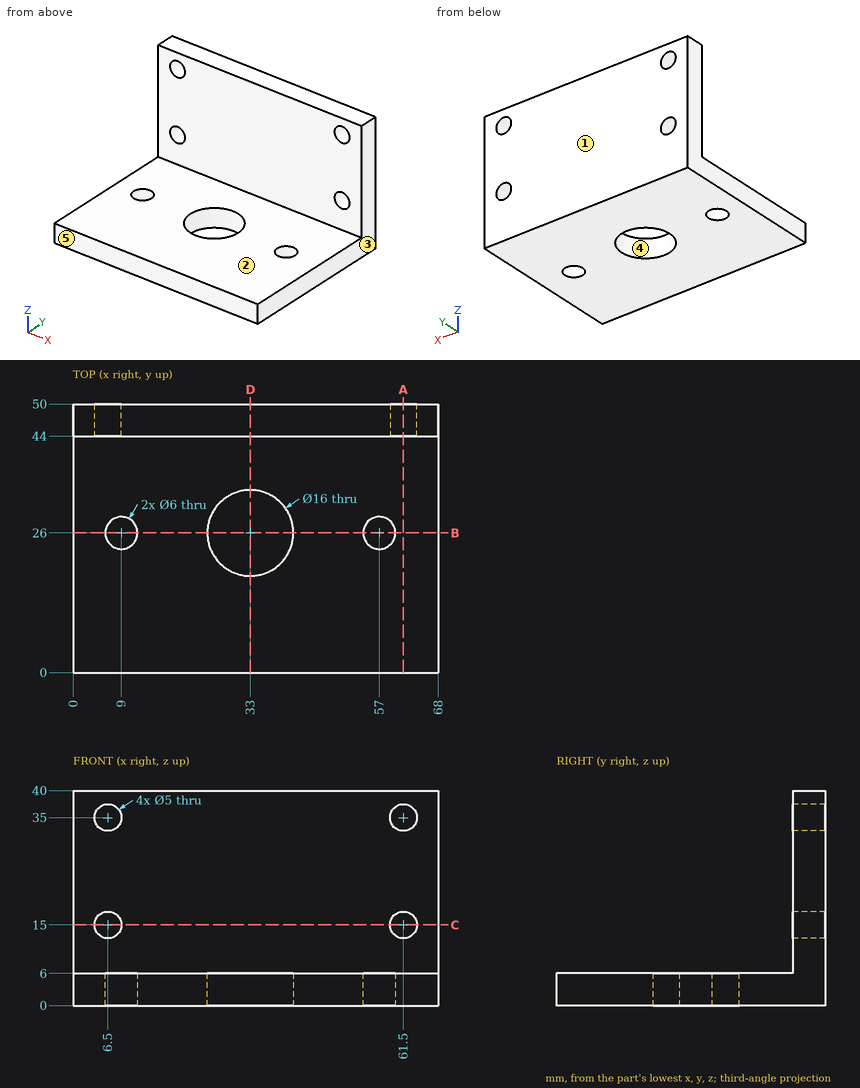
The drawing under review shows one solid part. Ordinate dimensions are in mm from its lowest x, y, z. A direction names the side the tool comes from. Give positions to 0.01 mm unless a question says otherwise; leave off trailing zeros. Order: outer loops, then holes, each group sorted by start corner. A loop starts at its lowest first (then second) coordinate and runs counter-clockwise, first axis right, second up. Notation, with made-up numbers: (68.25, 14.5) -> (122.25, 14.5) arc R33 ccw to (122.25, 44.5) -> close; hole circle Ø2 at (-7, -29.5). An arc over 180 degrees is marked (long way). Write item = value, one per line. Start each with the question number.
(1) For the marked faces 1 and 2, list the 3-axis set-ups (+Z, -Z, +X, -X, +Y, -Y) from which the entire face can be reached by the end or side of a thin tool; tool diameter is ignored.
(2) To check wall thickness, follow line 1 along X through (y, z) = (48.1, 15); line 2 along Y through (x, z) = (33, 1.5); line 3 along Z through (x, y) = (61, 47). State the ranges of each line that lie inside material, in increasing order.
(3) We need section D-D on x = 33. Write out the cut boundary in (y, z).
(4) We need section A-A on x = 61.5. Write out the cut boundary in (y, z), plus the area to 3 significant figures.
(5) We need section B-B on y = 26. Write out the cut boundary in (x, z), plus the area to 3 significant figures.
(6) For pin 1 (10 mm diameter, centred on x = 11.5, y = 35, fed in from +Z); pin 2 (17 mm diameter, centred on x = 48, z = 19.5, fed in from -Y), all flat-tipped, find the tip position at first contact; note any pin that passes through.
(7) Mouldability with a two-part tool opening along Y and no side actions: class the marked faces 3, 4 and 5 as +Y half, -Y half, draft (parallel to the pull), parting line (faces both ways), or undercut.
(8) We need section C-C on z = 15. Write out the cut boundary in (x, y).
Numbers:
q1.face_1 = +Z, -Z, +X, -X, +Y
q1.face_2 = +Z, +X, -X, -Y
q2.line_1 = 0 to 4, 9 to 59, 64 to 68
q2.line_2 = 0 to 18, 34 to 50
q2.line_3 = 0 to 12.55, 17.45 to 32.55, 37.45 to 40
q3.outline = (0, 0) -> (18, 0) -> (18, 6) -> (0, 6) -> close; (34, 0) -> (50, 0) -> (50, 40) -> (44, 40) -> (44, 6) -> (34, 6) -> close
q4.outline = (0, 0) -> (50, 0) -> (50, 12.5) -> (44, 12.5) -> (44, 6) -> (0, 6) -> close; (44, 17.5) -> (50, 17.5) -> (50, 32.5) -> (44, 32.5) -> close; (44, 37.5) -> (50, 37.5) -> (50, 40) -> (44, 40) -> close
q4.area = 444 mm^2
q5.outline = (0, 0) -> (6, 0) -> (6, 6) -> (0, 6) -> close; (12, 0) -> (25, 0) -> (25, 6) -> (12, 6) -> close; (41, 0) -> (54, 0) -> (54, 6) -> (41, 6) -> close; (60, 0) -> (68, 0) -> (68, 6) -> (60, 6) -> close
q5.area = 240 mm^2
q6.pin_1 = 6
q6.pin_2 = 44
q7.face_3 = draft
q7.face_4 = undercut
q7.face_5 = -Y half
q8.outline = (0, 44) -> (4, 44) -> (4, 50) -> (0, 50) -> close; (9, 44) -> (59, 44) -> (59, 50) -> (9, 50) -> close; (64, 44) -> (68, 44) -> (68, 50) -> (64, 50) -> close
